Autodesk Inventor part; units mm, degrees
ref_plane "YZ Plane" through (0, 0, 0) normal (1, 0, 0) x (0, 1, 0)
ref_plane "XZ Plane" through (0, 0, 0) normal (0, 1, 0) x (-1, 0, 0)
ref_plane "XY Plane" through (0, 0, 0) normal (0, 0, 1) x (1, 0, 0)
sketch "Sketch1" plane through (0, 0, 0) normal (0, 0, 1) x (1, 0, 0)
  line L0 (0, 0) -> (50, 0)
  line L1 (50, 0) -> (50, 50)
  line L2 (50, 50) -> (0, 0)
  dimension "d0" = 50
  dimension "d1" = 50
extrude "Extrusion1" add sketch "Sketch1" along normal blind 20
sketch "Sketch2" plane through (0, 0, 20) normal (0, 0, 1) x (1, 0, 0)
  line L0 (50, 50) -> (0, 0)
  line L1 (5, 5) -> (45, 5)
  line L2 (45, 5) -> (45, 45)
  line L3 (50, 0) -> (50, 50)
  line L4 (0, 0) -> (50, 0)
  dimension "d4" = 5
  dimension "d5" = 5
extrude "Extrusion2" cut sketch "Sketch2" against normal through all contours L2 L1 L0
extrude "Extrusion3" add sketch "Sketch2" against normal blind 5 contours L2 L1 L0
sketch "Sketch3" plane through (0, 0, 0) normal (0, 0, -1) x (-1, 0, 0)
  line L0 (-12.7, 0) -> (-50, 37.3)
  line L1 (-50, 0) -> (-50, 50)
  line L2 (-60.6675, 53.6604) -> (-50, 37.3)
  line L3 (-60.6675, 53.6604) -> (-37.4752, 61.571)
  line L4 (-37.4752, 61.571) -> (23.8314, -5.4888)
  line L5 (23.8314, -5.4888) -> (-5.9204, -12.6802)
  line L6 (-5.9204, -12.6802) -> (-12.7, 0)
  point P0 (0, 0)
  dimension "d12" = 12.7
  dimension "d13" = 12.7
extrude "Extrusion5" cut sketch "Sketch3" against normal through all
sketch "Sketch4" plane through (0, 0, 15) normal (0, 0, -1) x (-1, 0, 0)
  line L0 (-17.7, 5) -> (-45, 32.3)
  line L1 (-45, 5) -> (-45, 32.3)
  point P0 (0, 0)
  point P1 (-38, 12)
  dimension "d17" = 7
  dimension "d27" = 7
hole "Hole1" at (38, 12, 15) direction (0, 0, 1) diameter 8 depth 25.4 tip angle 118
sketch "Sketch5" plane through (45, 5, 0) normal (-1, 0, 0) x (0, 0, 1)
  line L0 (0, 0) -> (0, 27.3)
  line L1 (20, -5) -> (0, -5)
  point P0 (10, 22)
  point P1 (10, 7)
  dimension "d28" = 10
  dimension "d29" = 10
  dimension "d30" = 15
  dimension "d31" = 12
hole "Hole2" at (45, 27, 10) at (45, 12, 10) direction (1, 0, 0) diameter 5 depth 25.4 tip angle 118
sketch "Sketch6" plane through (45, 5, 15) normal (0, 1, 0) x (1, 0, 0)
  line L0 (-27.3, 15) -> (0, 15)
  line L1 (5, 15) -> (5, -5)
  point P0 (-45, 15)
  point P1 (-7, 5)
  point P2 (-22, 5)
  dimension "d39" = 15
  dimension "d40" = 10
  dimension "d41" = 10
  dimension "d42" = 12
hole "Hole3" at (38, 5, 10) at (23, 5, 10) direction (0, -1, 0) diameter 5 depth 25.4 tip angle 118
sketch "Sketch7" plane through (0, 0, 0) normal (0, 0, -1) x (-1, 0, 0)
  line L0 (-17.7, 5) -> (-17.7, 0)
  line L1 (-12.7, 0) -> (-50, 0)
  line L2 (-17.7, 0) -> (-12.7, 0)
  line L3 (-12.7, 0) -> (-17.7, 5)
  line L4 (-12.7, 0) -> (-17.7, 5)
  line L5 (-45, 32.3) -> (-50, 32.3)
  line L6 (-50, 0) -> (-50, 37.3)
  line L7 (-50, 32.3) -> (-50, 37.3)
  line L8 (-50, 37.3) -> (-45, 32.3)
  line L9 (-45, 32.3) -> (-50, 37.3)
  point P0 (0, 0)
extrude "Extrusion6" cut sketch "Sketch7" against normal blind 25.4
sketch "Sketch8" plane through (0, 0, 0) normal (0, 0, -1) x (-1, 0, 0)
  line L0 (-17.7, 0) -> (-50, 0)
  line L1 (-38, 0) -> (-60.6544, 0)
  line L2 (-60.6544, 0) -> (-60.6544, 37.4521)
  line L3 (-60.6544, 37.4521) -> (-38, 37.4521)
  line L4 (-38, 37.4521) -> (-38, 0)
  circle A0 centre (-38, 12) radius 4
  point P0 (0, 0)
  dimension "d52" = 0
extrude "Extrusion7" cut sketch "Sketch8" against normal through all contours L0 L1 L2 L3 L4 A0 | A0 L4 picked at (-39.3236, 12.1607)
mirror "Mirror1" about plane through (38, 37.4521, 0) normal (1, 0, 0)
sketch "Sketch9" plane through (0, 0, 15) normal (0, 0, -1) x (-1, 0, 0)
  point P0 (0, 0)
fillet "Fillet1" radius 8 1 edges at (38, 25.3, 17.5)
sketch "Sketch10" plane through (0, 0, 20) normal (0, 0, 1) x (1, 0, 0)
  arc A0 (9.2418, 17.7) -> (17.7, 5) centre (17.0156, 13.7108) ccw
  arc A1 (58.3, 5) -> (66.7582, 17.7) centre (58.9844, 13.7108) ccw
  arc A2 (66.7582, 17.7) -> (9.2418, 17.7) centre (38, 2.9422) ccw
  line L0 (17.7, 5) -> (32.3431, 19.6431)
  line L1 (32.3431, 19.6431) -> (17.7, 5)
  line L2 (58.3, 5) -> (43.6569, 19.6431)
  arc A3 (43.6569, 19.6431) -> (32.3431, 19.6431) centre (38, 13.9863) ccw
  line L3 (58.3, 5) -> (43.6569, 19.6431)
  arc A4 (43.6569, 19.6431) -> (32.3431, 19.6431) centre (38, 13.9863) ccw
  point P0 (0, 0)
  dimension "d56" = 8.7376
  dimension "d57" = 8.4582
  dimension "d58" = 12.7
  dimension "d59" = 12.7
  dimension "d60" = 8.4582
  dimension "d61" = 0
extrude "Extrusion8" add sketch "Sketch10" against normal up to surface (5 mm away)
sketch "Sketch12" plane through (0, 0, 20) normal (0, 0, 1) x (1, 0, 0)
  arc A0 (17.7, 16.5588) -> (17.7, 7.2332) centre (19.8547, 11.896) ccw
  line L0 (17.7, 16.5588) -> (31.0503, 23.6999)
  arc A1 (44.6361, 23.6999) -> (31.0503, 23.6999) centre (37.8432, 12.753) ccw
  line L1 (58.3, 5) -> (63.7675, 1.1638)
  line L2 (63.7675, 1.1638) -> (73.9162, 6.1166)
  line L3 (73.9162, 6.1166) -> (79.7366, 33.6983)
  line L4 (79.7366, 33.6983) -> (40.092, 40.6944)
  line L5 (40.092, 40.6944) -> (0, 39.3618)
  line L6 (0, 39.3618) -> (-15.8768, 5)
  arc A2 (-15.8768, 5) -> (-14.2095, 1.1638) centre (-13.3336, 3.8249) ccw
  line L7 (-14.2095, 1.1638) -> (10.6084, -22.6037)
  line L8 (10.6084, -22.6037) -> (17.7, 5)
  line L9 (17.7, 7.2332) -> (17.7, 5)
  line L10 (58.3, 7.7519) -> (58.3, 5)
  line L11 (44.6361, 23.6999) -> (58.3, 16.7272)
  arc A3 (58.3, 7.7519) -> (58.3, 16.7272) centre (56.2845, 12.2396) ccw
  point P0 (0, 0)
extrude "Extrusion9" cut sketch "Sketch12" against normal through all
sketch "Sketch13" plane through (0, 0, 20) normal (0, 0, 1) x (1, 0, 0)
  circle A0 centre (19.6322, 11.9106) radius 2.4728
  circle A1 centre (56.125, 12.2133) radius 2.4552
  point P0 (0, 0)
extrude "Extrusion10" cut sketch "Sketch13" against normal blind 25.4
sketch "Sketch14" plane through (17.7, 5, 15) normal (0, 1, 0) x (1, 0, 0)
  line L0 (26.9361, 0) -> (13.3503, 0)
  line L1 (10, 15) -> (15, 15)
  line L2 (15, 15) -> (15, 0)
  line L3 (15, 0) -> (10, 0)
  line L4 (10, 0) -> (10, 15)
  line L5 (40.6, 15) -> (0, 15)
  line L6 (25.6, 15) -> (30.6, 15)
  line L7 (30.6, 15) -> (30.6, 0)
  line L8 (30.6, 0) -> (25.6, 0)
  line L9 (25.6, 0) -> (25.6, 15)
  line L10 (40.6, 15) -> (40.6, 0)
  line L11 (0, 15) -> (0, 0)
  point P0 (-17.7, 15)
  dimension "d51" = 0
  dimension "d83" = 10
  dimension "d84" = 5
  dimension "d85" = 10
  dimension "d86" = 5
extrude "Extrusion11" add sketch "Sketch14" along normal blind 15 contours L0 L9 L5 L7 L8 | L0 L3 L4 L1 L2
chamfer "Chamfer1" distance 15 angle 45 2 edges at (45.8, 20, 0) (30.2, 20, 0)
sketch "Sketch15" plane through (58.3, 0, 0) normal (1, 0, 0) x (0, 0, -1)
  line L0 (-20, 7.7519) -> (-20, 0)
  line L1 (-20, 0) -> (0, 0)
  line L2 (0, 0) -> (0, 5)
  line L3 (0, 5) -> (-15, 5)
  line L4 (-15, 7.7519) -> (-15, 5)
  line L5 (-20, 7.7519) -> (-15, 7.7519)
  point P0 (0, 0)
extrude "Extrusion12" add sketch "Sketch15" along normal blind 3
sketch "Sketch16" plane through (17.7, 0, 0) normal (-1, 0, 0) x (0, 0, 1)
  line L0 (20, 7.2332) -> (20, 0)
  line L1 (20, 7.2332) -> (15, 7.2332)
  line L2 (15, 5) -> (15, 7.2332)
  line L3 (0, 5) -> (15, 5)
  line L4 (0, 0) -> (0, 5)
  line L5 (20, 0) -> (0, 0)
extrude "Extrusion13" add sketch "Sketch16" along normal blind 3
sketch "Sketch17" plane through (0, 0, 15) normal (0, 0, -1) x (-1, 0, 0)
  line L0 (-14.7, 7.2332) -> (-14.7181, 11.916)
  arc A0 (-17.7, 7.2332) -> (-17.7, 16.5588) centre (-19.8547, 11.896) ccw
  line L1 (-14.7181, 11.916) -> (-19.0926, 6.6114)
  line L2 (-19.0926, 6.6114) -> (-14.7, 7.2332)
  line L3 (-61.3, 7.7519) -> (-61.2028, 12.3437)
  arc A1 (-58.3, 16.7272) -> (-58.3, 7.7519) centre (-56.2845, 12.2396) ccw
  line L4 (-61.2028, 12.3437) -> (-58.3, 7.7519)
  line L5 (-58.3, 7.7519) -> (-58.6002, 6.2246)
  line L6 (-58.6002, 6.2246) -> (-61.3, 7.7519)
  point P0 (0, 0)
extrude "Extrusion14" add sketch "Sketch17" against normal up to surface (5 mm away) contours L2 L1 L0 | L3 A1 L5 L6
properties part number "Leadscrew Mount"
Input: part model. Units: mm. Frame: model coordinates. A direction names the side the tool comes from. Give positions to 0.01 mm unless a question says otherwise; leave off trailing zeros. Loops run counter-clockwise (first coordinate to the right, second up) from the corner with the lowest first, then second, coordinate; pieces in that order, holes last. Notation, with made-up numbers: (17, 43.5) - (23, 43.5) arc R18 cw to (23, 55.5) - close; hole circle Ø5 at (-25, 81.25). An arc over 180 degrees is marked (long way). Use CSV: the item, a comma, the result in double quotes. Start each with the question number.
Item 1: Reachability of faces 4 (the flat face through (27.7, 11, 9)), 5 (the flat face through (32.7, 11, 9)), 6 (the flat face through (51.372, 20.262, 17.535)), 7 (the cylindrical face through (58.467, 12.951, 17.535)), 8 (the flat face through (48.3, 11, 9)) from +Z, -Z, +X, -X, +Y, -Y: full face, straight path, thin tool, end or side. Return the list, or none.
Item 2: Line query: line 1 (X direction, y = 3.85, z = 10); line 2 (X direction, y = 12, z = 18.55); line 3 (Y direction, x = 31, z = 11). Output: solid intervals per line, ascending.
Item 3: Section C-C on y = 4.25. Return loops of the section in (x, z), then the cut area to 3 significant figures.
Item 4: Contact query for flat-ended pins moving along their axis: P1, Ø6, axis at x = 29.5, y = 19.5, coming from the -Z side; P2, Ø5, axis at y = 14.5, z = 8.5, coming from the -X side; P3, Ø9, axis at x = 38, y = 12, coming from the -Z side; P4, Ø1, axis at x = 56.5, z = 9.5, coming from the -Y side. Output: stop coordinate, or through.
Item 5: Section B-B on x = 52.5. Return loops of the section in (y, z), then the cut area to 3 significant figures.
Item 6: Section A-A on z = 10. Return loops of the section in (x, y), then the cut area to 3 significant figures.
Item 7: Section D-D on x = 38. Return loops of the section in (y, z).
Item 8: Mould query, pull axis X, two halves, no side actions, for faces 1 (the flat face through (14.7, 3, 10)), 2 (the flat face through (30, 13, 8)), 3 (the flat face through (36.7, 5, 7.6)). Classes: pulls with the +X half, pulls with the -X half, needs draft (parallel to the pull), parting line crosses it, or undercut.
Ans:
1,face 4,"-Z, -X, +Y"
1,face 5,"-Z, +Y"
1,face 6,"+Z, -Z, +X, +Y"
1,face 7,"+Z, -Z"
1,face 8,"-Z, +X, +Y"
2,line 1,"x = 14.7 to 20.5, 25.5 to 35.5, 40.5 to 50.5, 55.5 to 61.3"
2,line 2,"x = 14.72 to 17.16, 22.1 to 34, 42 to 53.68, 58.57 to 61.21"
2,line 3,"y = 0 to 16"
3,outline,"(14.7, 0) - (61.3, 0) - (61.3, 20) - (14.7, 20) - close; hole circle Ø5 at (23, 10); hole circle Ø5 at (38, 10); hole circle Ø5 at (53, 10)"
3,area,"873 mm2"
4,P1,"stops at z = 11.5"
4,P2,"stops at x = 27.7"
4,P3,"stops at z = 15"
4,P4,"stops at y = 0"
5,outline,"(0, 0) - (5, 0) - (5, 7.55) - (0, 7.55) - close; (0, 12.45) - (5, 12.45) - (5, 15) - (19.69, 15) - (19.69, 20) - (0, 20) - close"
5,area,"149 mm2"
6,outline,"(14.7, 0) - (20.5, 0) - (20.5, 5) - (14.7, 5) - close; (25.5, 0) - (35.5, 0) - (35.5, 5) - (32.7, 5) - (32.7, 15) - (27.7, 15) - (27.7, 5) - (25.5, 5) - close; (40.5, 0) - (50.5, 0) - (50.5, 5) - (48.3, 5) - (48.3, 15) - (43.3, 15) - (43.3, 5) - (40.5, 5) - close; (55.5, 0) - (61.3, 0) - (61.3, 5) - (55.5, 5) - close"
6,area,"258 mm2"
7,outline,"(0, 0) - (5, 0) - (5, 7.5) - (0, 7.5) - close; (0, 12.5) - (5, 12.5) - (5, 15) - (8, 15) - (8, 20) - (0, 20) - close; (16, 15) - (25.64, 15) - (25.64, 20) - (16, 20) - close"
8,face 1,"pulls with the -X half"
8,face 2,"needs draft"
8,face 3,"undercut"
